Autodesk Inventor part; units mm, degrees
ref_plane "YZ Plane" through (0, 0, 0) normal (1, 0, 0) x (0, 1, 0)
ref_plane "XY Plane" through (0, 0, 0) normal (0, 0, 1) x (1, 0, 0)
sketch "Sketch1" plane through (0, 0, 0) normal (1, 0, 0) x (0, 1, 0)
  circle A0 centre (0, 0) radius 3
  circle A1 centre (0, 0) radius 70
  dimension "d0" = 140
  dimension "d1" = 6
extrude "Extrusion1" add sketch "Sketch1" along normal blind 10
fillet "Fillet1" radius 2 2 edges at (10, -70, 0) (0, -70, 0)
sketch "Sketch2" plane through (10, 0, 0) normal (1, 0, 0) x (0, 0, -1)
  circle A0 centre (0, 40) radius 10
  circle A1 centre (0, 0) radius 3
  dimension "d5" = 20
  dimension "d6" = 40
extrude "Extrusion2" cut sketch "Sketch2" against normal blind 10 contours A0
pattern_circular "Circular Pattern1" count 6 over 360 about axis through (0, 0, 0) along (1, 0, 0) of "Extrusion2"
ref_plane "Work Plane1" through (0, -70, 0) normal (0, 1, 0) x (-1, 0, 0)
properties part number "05_Banh_xe" material "Acetal Resin, Black"
Geometry: final body of the model. Coordinates: model frame, mm. Give positions to 0.01 mm unless a question says otherwise; leave off trailing zeros. Write each loop counter-clockwise with the first axis right and the second up, starting at its lowest first coordinate (ties: lowest second). Pieces come first, ordered by that corner, then holes.
1. Section query B-B, the plane z = 0. Return loops of the section in (x, y), then the cut area to 3 significant figures.
2. Draft query along Y for faces 1 (the cylindrical face through (4.958, -55.55, 42.594)), 2 (the flat face through (0, -1, -14)), 3 (the cylindrical face through (5.07, -13.24, 42.01)). Return one class per face: released by +Y, released by -Y, zero draft, split by the parting line, or undercut.
3. Section query A-A, the plane y = 0. Return loops of the section in (x, z), then the cut area to 3 significant figures.
4. Line query: probe 1 along Y at (x, z) = (9.25, -4); probe 2 along Z at (x, y) = (4, 23); probe 3 along Z at (x, y) = (5.5, -11). Output: solid intervals per line, ascending.
5. Pin query (flat end, axial travel): P1, Ø12, axis at y = -40, z = 0, coming from the -X side; P2, Ø3, axis at x = 8.5, y = -46.5, coming from the -Z side; P3, Ø1.5, axis at x = 3, y = -15, coming from the +Z side; P4, Ø4, axis at x = 7.5, z = 25, coming from the +Y side. Return the tip coordinate at first contact, or that it passes through.
6. Section query C-C, the plane x = 6. Return loops of the section in (y, z), then the cut area to 3 significant figures.
7. Section query D-D, the plane z = 42.5. Count the separate pieces of the cut face and the enclosed holes in it, then the cut area to 3 significant figures.
Computed:
1. outline: (0, -68) arc R2 ccw to (2, -70) - (8, -70) arc R2 ccw to (10, -68) - (10, -50) - (0, -50) - close; (0, -30) - (10, -30) - (10, -3) - (0, -3) - close; (0, 3) - (10, 3) - (10, 30) - (0, 30) - close; (0, 50) - (10, 50) - (10, 68) arc R2 ccw to (8, 70) - (2, 70) arc R2 ccw to (0, 68) - close
1. area: 937 mm2
2. face 1: split by the parting line
2. face 2: zero draft
2. face 3: undercut
3. outline: (0, -68) arc R2 ccw to (2, -70) - (8, -70) arc R2 ccw to (10, -68) - (10, -3) - (0, -3) - close; (0, 3) - (10, 3) - (10, 68) arc R2 ccw to (8, 70) - (2, 70) arc R2 ccw to (0, 68) - close
3. area: 1,340 mm2
4. probe 1: y = -69.45 to -49.17, -30.83 to 30.83, 49.17 to 69.45
4. probe 2: z = -66.11 to -44.18, -25.1 to 25.1, 44.18 to 66.11
4. probe 3: z = -69.13 to -39, -30.28 to 30.28, 39 to 69.13
5. P1: passes through
5. P2: stops at z = -53.58
5. P3: stops at z = 68.53
5. P4: stops at y = 66.11
6. outline: circle Ø140 at (0, 0); hole circle Ø20 at (-40, 0); hole circle Ø20 at (-20, -34.64); hole circle Ø20 at (-20, 34.64); hole circle Ø6 at (0, 0); hole circle Ø20 at (20, -34.64); hole circle Ø20 at (20, 34.64); hole circle Ø20 at (40, 0)
6. area: 13,500 mm2
7. separate pieces: 3
7. enclosed holes: 0
7. area: 861 mm2
